Source: CAD feature listing. Evaluate the final solid. Frame: model axes, mm. Face numbers are marked on the shaded views. A direction names the side the tool comes from. Coordinates: 2 decimals unless noted, no trailing zeros. Loops run counter-clockwise (first coordinate to the right, second up) from the corner with the lowest first, then second, coordinate; pieces in that order, holes last.
Item 1: Section query D-D, the plane z = -3. Return the cut outline in (x, y), then the cut area to 3 significant figures.
Item 2: Section query A-A, the plane x = -7.25. Return the cut outline in (y, z) (3 decimals).
Item 3: Section query B-B, the plane z = -12. Return the cut outline in (x, y).
Item 4: Section query C-C, the plane y = -0.4. Return the cut outline in (x, z), then the cut area to 3 significant figures.
Item 5: Line query: probe 1 along Y at (x, z) = (-8.5, -10.75); probe 2 along Z at (x, y) = (-7.75, -3.7); probe 3 along X at (y, z) = (-0.45, -16.25). Output: solid intervals per line, ascending.
Item 6: Reachability of the marked faces 1, 2, 3 and 4 from +Z, -Z, +X, -X, +Y, -Y: full face, straight path, thin tool, end or side. Return the list, or none.
Item 7: Pin query (flat end, axial travel): pin 1 Ø1.4 at (x, y) = (-4.5, -3) entering from +Z; pin 2 Ø3 at (x, z) = (-5, -11) entering from -Y; pin 3 Ø2.5 at (y, z) = (-2, -8.5) entering from +X; pin 4 Ø2 at (y, z) = (-4, -14) entering from +X. Return the tip coordinate at first contact, or that it passes through.
Autodesk Inventor part; units mm, degrees
ref_plane "YZ Plane" through (0, 0, 0) normal (1, 0, 0) x (0, 1, 0)
ref_plane "XZ Plane" through (0, 0, 0) normal (0, 1, 0) x (-1, 0, 0)
ref_plane "XY Plane" through (0, 0, 0) normal (0, 0, 1) x (1, 0, 0)
sketch "Sketch1" plane through (0, 0, 0) normal (0, 1, 0) x (-1, 0, 0)
  line L0 (0, 0) -> (10.16, 0)
  line L1 (10.16, 0) -> (10.16, -23.495)
  line L2 (10.16, -23.495) -> (0, -23.495)
  line L3 (0, -23.495) -> (0, 0)
  line L4 (8.001, -21.336) -> (8.001, -2.159)
  line L5 (8.001, -2.159) -> (2.159, -2.159)
  line L6 (2.159, -2.159) -> (2.159, -21.336)
  line L7 (2.159, -21.336) -> (8.001, -21.336)
  dimension "d0" = 23.495
  dimension "d1" = 10.16
  dimension "d2" = 2.159
extrude "Extrusion1" add sketch "Sketch1" along normal blind 1.016 contours L0 L1 L2 L3 | L7 L6 L5 L4
extrude "Extrusion2" add sketch "Sketch1" against normal blind 1.016 contours L7 L6 L5 L4
fillet "Fillet1" radius 1.27 4 edges at (0, 0.508, 0) (0, 0.508, -23.495) (-10.16, 0.508, -23.495) (-10.16, 0.508, 0)
sketch "Sketch2" plane through (0, -1.016, 0) normal (0, -1, 0) x (1, 0, 0)
  line L0 (-8.001, -2.159) -> (-8.001, -21.336)
  line L1 (-8.001, -21.336) -> (-2.159, -21.336)
  line L2 (-2.159, -21.336) -> (-2.159, -2.159)
  line L3 (-2.159, -2.159) -> (-8.001, -2.159)
  line L4 (-2.159, -4.699) -> (-8.001, -4.699)
  point P0 (0, 0)
  dimension "d8" = 2.54
extrude "Extrusion3" add sketch "Sketch2" along normal blind 3.81 contours L3 L2 L4 L0
properties part number "HallEffectSensorCaseLid" material "ABS Plastic"
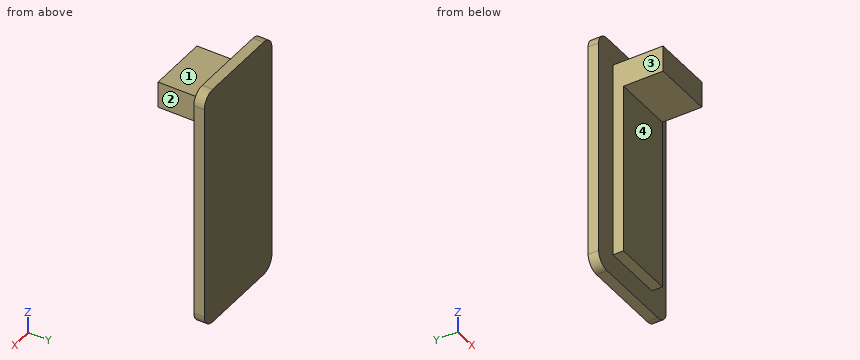
Verdict:
1. outline: (-10.16, 0) - (-8, 0) - (-8, -4.83) - (-2.16, -4.83) - (-2.16, 0) - (0, 0) - (0, 1.02) - (-10.16, 1.02) - close
1. area: 38.5 mm2
2. outline: (-4.826, -4.699) - (-1.016, -4.699) - (-1.016, -21.336) - (0, -21.336) - (0, -23.495) - (1.016, -23.495) - (1.016, 0) - (0, 0) - (0, -2.159) - (-4.826, -2.159) - close
3. outline: (-10.16, 0) - (-8, 0) - (-8, -1.02) - (-2.16, -1.02) - (-2.16, 0) - (0, 0) - (0, 1.02) - (-10.16, 1.02) - close
4. outline: (-8, -21.34) - (-2.16, -21.34) - (-2.16, -2.16) - (-8, -2.16) - close
4. area: 112 mm2
5. probe 1: y = 0 to 1.02
5. probe 2: z = -4.7 to -2.16
5. probe 3: x = -8 to -2.16
6. face 1: +Z, +X, -X, -Y
6. face 2: +Z, -Z, +X, -Y
6. face 3: +Z, -Z, -X, -Y
6. face 4: -Z, +X, -X, -Y
7. pin 1: stops at z = -2.16
7. pin 2: stops at y = -1.02
7. pin 3: stops at x = -2.16
7. pin 4: passes through
